```python
from build123d import *

# Parameters (mm, degrees)
SKETCH_1_R          = 26
EXTRUDE_1_DEPTH     = 4
SKETCH_2_R          = 4.75
EXTRUDE_2_DEPTH     = 20
SKETCH_3_R          = 3
CUT_EXTRUDE_1_DEPTH = 20
SKETCH_4_R          = 26
SKETCH_4_R_2        = 23
EXTRUDE_3_DEPTH     = 18
CUT_EXTRUDE_2_DEPTH = 5
SKETCH_6_R          = 5
CUT_EXTRUDE_3_DEPTH = 2
SKETCH_7_R          = 2.5
EXTRUDE_4_DEPTH     = 3


with BuildPart() as part:
    # 草图1 → 凸台-拉伸1 (new body)
    with BuildSketch(Plane(origin=(0, 0, 0), x_dir=(0, 0, -1), z_dir=(1, 0, 0))):
        Circle(SKETCH_1_R)
    extrude(amount=EXTRUDE_1_DEPTH)

    # 草图2 → 凸台-拉伸2 (add)
    with BuildSketch(Plane(origin=(4, 0, 0), x_dir=(0, 0, -1), z_dir=(1, 0, 0))):
        Circle(SKETCH_2_R)
    extrude(amount=EXTRUDE_2_DEPTH)

    # 草图3 → 切除-拉伸1 (cut)
    with BuildSketch(Plane(origin=(24, 0, 0), x_dir=(0, 0, -1), z_dir=(1, 0, 0))):
        Circle(SKETCH_3_R)
    extrude(amount=-CUT_EXTRUDE_1_DEPTH, mode=Mode.SUBTRACT)

    # 草图4 → 凸台-拉伸3 (add)
    with BuildSketch(Plane(origin=(4, 0, 0), x_dir=(0, 0, -1), z_dir=(1, 0, 0))):
        Circle(SKETCH_4_R)
        Circle(SKETCH_4_R_2, mode=Mode.SUBTRACT)
    extrude(amount=EXTRUDE_3_DEPTH)

    # 草图5 → 切除-拉伸2 (cut, through all)
    with BuildSketch(Plane(origin=(4, 0, 0), x_dir=(0, 0, -1), z_dir=(1, 0, 0))):
        with BuildLine():
            Line((-21.275079931, 8.739048799), (-4.408389392, 6.067627458))
            Line((-4.408389392, 6.067627458), (-1.736968051, 22.934317997))
            ThreePointArc((-1.736968051, 22.934317997), (-13.519060803, 18.607390871), (-21.275079931, 8.739048799))
        make_face()
        with BuildLine():
            Line((21.275079931, 8.739048799), (4.408389392, 6.067627458))
            Line((4.408389392, 6.067627458), (1.736968051, 22.934317997))
            ThreePointArc((1.736968051, 22.934317997), (13.519060803, 18.607390871), (21.275079931, 8.739048799))
        make_face()
        with BuildLine():
            Line((14.885690562, -17.53328881), (7.132923872, -2.317627458))
            Line((7.132923872, -2.317627458), (22.348585224, 5.435139232))
            ThreePointArc((22.348585224, 5.435139232), (21.874299875, -7.107390871), (14.885690562, -17.53328881))
        make_face()
        with BuildLine():
            Line((-12.075217218, -19.575217218), (0, -7.5))
            Line((0, -7.5), (12.075217218, -19.575217218))
            ThreePointArc((12.075217218, -19.575217218), (0, -23), (-12.075217218, -19.575217218))
        make_face()
        with BuildLine():
            Line((-22.348585224, 5.435139232), (-7.132923872, -2.317627458))
            Line((-7.132923872, -2.317627458), (-14.885690562, -17.53328881))
            ThreePointArc((-14.885690562, -17.53328881), (-21.874299875, -7.107390871), (-22.348585224, 5.435139232))
        make_face()
    extrude(amount=-CUT_EXTRUDE_2_DEPTH, mode=Mode.SUBTRACT)

    # 草图6 → 切除-拉伸3 (cut)
    with BuildSketch(Plane.ZY):
        Circle(SKETCH_6_R)
    extrude(amount=-CUT_EXTRUDE_3_DEPTH, mode=Mode.SUBTRACT)

    # 草图7 → 凸台-拉伸4 (add)
    with BuildSketch(Plane.ZY.offset(-2)):
        Circle(SKETCH_7_R)
    extrude(amount=EXTRUDE_4_DEPTH)


solid = part.part
```
Geometry check sheet. Reference: the model listing, model coordinates, mm. A direction names the side the tool comes from. Coordinates: 2 decimals unless noted, no trailing zeros. Order: outer loops, then holes, each group sorted by start corner. A loop starts at its lowest first (then second) coordinate and runs counter-clockwise, first axis right, second up.
Item 1: Section check C-C (z = -16). Enter the section's corners in (x, y).
Item 2: Section check D-D (x = 8.25). Enter the section's corners in (y, z).
Item 3: Tool access check on faces 1 (the flat face through (2, -2, 2)), 2 (the flat face through (2.028, -10.032, -11.064)), 3 (the flat face through (4, 0, 0)), 4 (the flat face through (24, -1, -3)). Record the directions out of +Z, -Z, +X, -X, +Y, -Y that give a thin tool (end or side, any length) a straight path to the whole face; none if there is none.
Item 4: Section check B-B (y = -4). Enter the section's corners in (x, z), plus the area to 3 significant figures.
Item 5: Scan lines: line 1 along Y through (x, z) = (9.75, 0); line 2 along Y through (x, z) = (10, -4); line 3 along Y through (x, z) = (3.75, 12.5). Record each from-to range of solid material in increasing order.
Item 6: Mould release check, pull along Z, two halves, no side actions. Record for faces 5 (the flat face through (2.028, 1.613, 14.847)), 6 (the flat face through (22, -21, -10)), 7 (the cylindrical face through (10.846, -15.821, 20.633)): released by +Z, released by -Z, zero draft, split by the parting line, or undercut.
Item 7: Depth check by flat-ended pin: pin 1 (4 mm diameter, centred on x = 2.5, z = 16.5, fed in from +Y); pin 2 (3 mm diameter, centred on x = 6, y = 13, fed in from +Z); pin 3 (3 mm diameter, centred on x = 20, z = 12, fed in from +Y). Enter the tip coordinate at first touch or a pass-through.
Item 8: Section check A-A (x = 0.75). Enter the section's corners in (y, z).
Check sheet entries:
1. outline: (0, -20.49) - (22, -20.49) - (22, -16.52) - (0, -16.52) - close; (0, 2.2) - (4, 2.2) - (4, 7.9) - (0, 7.9) - close; (0, 16.52) - (22, 16.52) - (22, 20.49) - (0, 20.49) - close
2. outline: circle Ø52 at (0, 0); circle Ø9.5 at (0, 0); hole circle Ø46 at (0, 0); hole circle Ø6 at (0, 0)
3. face 1: -X
3. face 2: +X, -X
3. face 3: +X
3. face 4: +Z, -Z, +X, +Y, -Y
4. outline: (0, -25.69) - (22, -25.69) - (22, -22.65) - (0, -22.65) - close; (0, -7.99) - (4, -7.99) - (4, -2.56) - (24, -2.56) - (24, 2.56) - (4, 2.56) - (4, 7.99) - (0, 7.99) - (0, 3) - (2, 3) - (2, -3) - (0, -3) - close; (0, 22.65) - (22, 22.65) - (22, 25.69) - (0, 25.69) - close
4. area: 288 mm2
5. line 1: y = -26 to -23, -4.75 to -3, 3 to 4.75, 23 to 26
5. line 2: y = -25.69 to -22.65, -2.56 to 2.56, 22.65 to 25.69
5. line 3: y = -22.8 to -12.85, 0.42 to 7.35, 19.31 to 22.8
6. face 5: undercut
6. face 6: zero draft
6. face 7: split by the parting line
7. pin 1: stops at y = 21.58
7. pin 2: stops at z = 23.32
7. pin 3: stops at y = 23.79
8. outline: circle Ø52 at (0, 0); circle Ø5 at (0, 0); hole (-19.58, -12.08) - (-7.5, 0) - (-19.58, 12.08) arc R23 ccw to start; hole (-17.53, -14.89) arc R23 ccw to (5.44, -22.35) - (-2.32, -7.13) - close; hole (-17.53, 14.89) - (-2.32, 7.13) - (5.44, 22.35) arc R23 ccw to start; hole circle Ø10 at (0, 0); hole (6.07, -4.41) - (8.74, -21.28) arc R23 ccw to (22.93, -1.74) - close; hole (6.07, 4.41) - (22.93, 1.74) arc R23 ccw to (8.74, 21.28) - close
